```python
from build123d import *

# Parameters (mm, degrees)
SKETCH_1_R               = 5
EXTRUDE_1_DEPTH          = 78
HOLE_WIZARD_M5_1_D       = 4.2
HOLE_WIZARD_M5_1_DEPTH   = 12.4
HOLE_WIZARD_M5_1_TIP     = 1.2618073
HOLE_WIZARD_M5_2_D       = 4.2
HOLE_WIZARD_M5_2_DEPTH   = 12.4
HOLE_WIZARD_M5_2_TIP     = 1.2618073
CUT_EXTRUDE_1_DEPTH      = 8
CUT_EXTRUDE_1_DEPTH_BACK = 8
SKETCH_6_W               = 7.505950336
SKETCH_6_H               = 7.971260953
SKETCH_6_W_2             = 6.842029893
SKETCH_6_H_2             = 4.427384225
SKETCH_6_W_3             = 6.476020113
SKETCH_6_H_3             = 7.384230107
SKETCH_6_W_4             = 6.951681063
SKETCH_6_H_4             = 4.627406651


with BuildPart() as part:
    # 草图1 → 凸台-拉伸1 (new body)
    with BuildSketch(Plane.XY):
        Circle(SKETCH_1_R)
    extrude(amount=EXTRUDE_1_DEPTH)

    # M5 螺纹孔1
    with Locations(Plane.XY.offset(78)):
        with Locations((0, 0)):
            Hole(HOLE_WIZARD_M5_1_D / 2, depth=HOLE_WIZARD_M5_1_DEPTH)
            with Locations((0, 0, -(HOLE_WIZARD_M5_1_DEPTH + HOLE_WIZARD_M5_1_TIP / 2))):  # 118° drill point
                Cone(0, HOLE_WIZARD_M5_1_D / 2, HOLE_WIZARD_M5_1_TIP, mode=Mode.SUBTRACT)

    # M5 螺纹孔2
    with Locations(Plane(origin=(0, 0, 0), x_dir=(-1, 0, 0), z_dir=(0, 0, -1))):
        with Locations((0, 0)):
            Hole(HOLE_WIZARD_M5_2_D / 2, depth=HOLE_WIZARD_M5_2_DEPTH)
            with Locations((0, 0, -(HOLE_WIZARD_M5_2_DEPTH + HOLE_WIZARD_M5_2_TIP / 2))):  # 118° drill point
                Cone(0, HOLE_WIZARD_M5_2_D / 2, HOLE_WIZARD_M5_2_TIP, mode=Mode.SUBTRACT)

    # 草图6 → 切除-拉伸1 (cut, two sides: drawn at the far end of the back side and taken through both)
    with BuildSketch(Plane.XY.offset(38).offset(-CUT_EXTRUDE_1_DEPTH_BACK)):
        with Locations((-7.952975168, -0.439871177)):
            Rectangle(SKETCH_6_W, SKETCH_6_H)
        with Locations((0.010635023, 6.413692112)):
            Rectangle(SKETCH_6_W_2, SKETCH_6_H_2)
        with Locations((7.438010056, -0.146355753)):
            Rectangle(SKETCH_6_W_3, SKETCH_6_H_3)
        with Locations((-0.075086924, -6.513703325)):
            Rectangle(SKETCH_6_W_4, SKETCH_6_H_4)
    extrude(amount=CUT_EXTRUDE_1_DEPTH + CUT_EXTRUDE_1_DEPTH_BACK, mode=Mode.SUBTRACT)


solid = part.part
```
Here's how the part is built. I have some questions about the finished solid (model axes, mm). A direction names the side the tool comes from. Give positions to 0.01 mm unless a question says otherwise; leave off trailing zeros. Order: outer loops, then holes, each group sorted by start corner. A loop starts at its lowest first (then second) coordinate and runs counter-clockwise, first axis right, second up. Notation, with made-up numbers: (47, 87.5) - (94, 87.5) arc R6 cw to (94, 95.5) - close; hole circle Ø7 at (59, 62). An arc over 180 degrees is marked (long way). Answer as a JSON object with one key per item and string values. Group by question number.
Item 1: If we mould it in two halves opening along X, with no side actions, what happens to faces 1 (the flat face through (4.2, 0, 38)), 2 (the flat face through (0, -4.2, 38)), 3 (the cylindrical face through (2.003, 0.631, 6.287))? For each: pulls with the +X half, pulls with the -X half, needs draft (parallel to the pull), parting line crosses it, or undercut.
Item 2: Which directions (+Z, -Z, +X, -X, +Y, -Y) give clear straight access to the entire face, cutting with the end or side of a thin tool? Please do faces 4 (the flat face through (1, -2.2, 0)), 5 (the flat face through (-4.2, 0, 38)), 6 (the flat face through (1, -2.2, 78)), 7 (the cylindrical face through (-2.003, 0.631, 71.713)), 8 (the flat face through (0, 4.2, 38)).
Item 3: Please list where these lines run through material, in increasing order: probe 1 along Y at (x, z) = (0, 7.5); probe 2 along X at (y, z) = (-1.5, 45).
Item 4: For P1, Ø1.6, axis at x = -1.5, z = 35, coming from the -Y side; P2, Ø2.5, axis at y = -1.5, z = 40.5, coming from the -X side; P3, Ø2.5, axis at y = 1, z = 41.5, coming from the +X side; P4, Ø1, axis at x = -1.5, y = 3, coming from the -Z side, each with a flat end and sliding along its axis, tell me the tip position at first contact or that it passes through.
Item 5: If we section it at A-A on z = 37.5: Please give me the cut outline in (x, y).
Item 6: If we section it at B-B on z = 67: Please give me the cut outline in (x, y).
Item 7: If we section it at C-C on z = 47: Please give me the cut outline in (x, y), and give its area (3 significant figures).
Result set:
{
 "1": {"face 1": "pulls with the +X half", "face 2": "needs draft", "face 3": "undercut"},
 "2": {"face 4": "-Z, +X, -X, +Y, -Y", "face 5": "-X, +Y, -Y", "face 6": "+Z, +X, -X, +Y, -Y", "face 7": "+Z", "face 8": "+X, -X, +Y"},
 "3": {"probe 1": "-5 to -2.1, 2.1 to 5", "probe 2": "-4.2 to 4.2"},
 "4": {"P1": "y = -4.2", "P2": "x = -4.2", "P3": "x = 4.2", "P4": "z = 0"},
 "5": {"outline": "(-4.2, -2.71) arc R5 ccw to (-2.71, -4.2) - (2.71, -4.2) arc R5 ccw to (4.2, -2.71) - (4.2, 2.71) arc R5 ccw to (2.71, 4.2) - (-2.71, 4.2) arc R5 ccw to (-4.2, 2.71) - close"},
 "6": {"outline": "circle Ø10 at (0, 0); hole circle Ø4.2 at (0, 0)"},
 "7": {"outline": "circle Ø10 at (0, 0)", "area": "78.5 mm²"}
}
